```python
from build123d import *

# Parameters (mm, degrees)
SKETCH_1_W             = 25
SKETCH_1_H             = 12
EXTRUDE_1_DEPTH        = 3
SKETCH_2_W             = 8
SKETCH_2_H             = 12
EXTRUDE_2_DEPTH        = 3
FILLET_1_R             = 3
FILLET_2_R             = 1.5
SKETCH_3_R             = 1.6
CUT_EXTRUDE_1_DEPTH    = 3
FILLET_1_OF_MIRROR_1_R = 3
FILLET_2_OF_MIRROR_1_R = 1.5
SKETCH_4_R             = 1.6
CUT_EXTRUDE_2_DEPTH    = 3


with BuildPart() as part:
    # 草图1 → 凸台-拉伸1 (new body)
    with BuildSketch(Plane.XY):
        with Locations((0, -24)):
            Rectangle(SKETCH_1_W, SKETCH_1_H)
    extrude(amount=EXTRUDE_1_DEPTH)

    # 草图2 → 凸台-拉伸2 (add)
    with BuildSketch(Plane.ZY.offset(12.5)):
        with Locations((7, -24)):
            Rectangle(SKETCH_2_W, SKETCH_2_H)
    extrude_2 = extrude(amount=-EXTRUDE_2_DEPTH)

    # 圆角1
    fillet_1_edges = [part.edges().sort_by_distance(p)[0] for p in [
        (-11, -18, 11),
        (-11, -30, 11),
    ]]
    fillet(fillet_1_edges, radius=FILLET_1_R)

    # 圆角2
    fillet_2_edges = [part.edges().sort_by_distance(p)[0] for p in [
        (-9.5, -24, 3),
    ]]
    fillet(fillet_2_edges, radius=FILLET_2_R)

    # 草图3 → 切除-拉伸1 (cut)
    with BuildSketch(Plane.ZY.offset(12.5)):
        with Locations(Location((7, -24, 0), (0, 0, 270))):
            Circle(SKETCH_3_R)
    cut_extrude_1 = extrude(amount=-CUT_EXTRUDE_1_DEPTH, mode=Mode.SUBTRACT)

    # 镜向1: 凸台-拉伸2, 切除-拉伸1 across plane
    add(extrude_2.mirror(Plane(origin=(0, 0, 0), x_dir=(0, 0, 1), z_dir=(1, 0, 0))))
    add(cut_extrude_1.mirror(Plane(origin=(0, 0, 0), x_dir=(0, 0, 1), z_dir=(1, 0, 0))), mode=Mode.SUBTRACT)

    # 圆角1 of 镜向1
    fillet_1_of_mirror_1_edges = [part.edges().sort_by_distance(p)[0] for p in [
        (11, -18, 11),
        (11, -30, 11),
    ]]
    fillet(fillet_1_of_mirror_1_edges, radius=FILLET_1_OF_MIRROR_1_R)

    # 圆角2 of 镜向1
    fillet_2_of_mirror_1_edges = [part.edges().sort_by_distance(p)[0] for p in [
        (9.5, -24, 3),
    ]]
    fillet(fillet_2_of_mirror_1_edges, radius=FILLET_2_OF_MIRROR_1_R)

    # 草图4 → 切除-拉伸2 (cut)
    with BuildSketch(Plane.XY.offset(3)):
        with Locations((5, -24)):
            Circle(SKETCH_4_R)
        with Locations((-5, -24)):
            Circle(SKETCH_4_R)
    extrude(amount=-CUT_EXTRUDE_2_DEPTH, mode=Mode.SUBTRACT)


solid = part.part
```
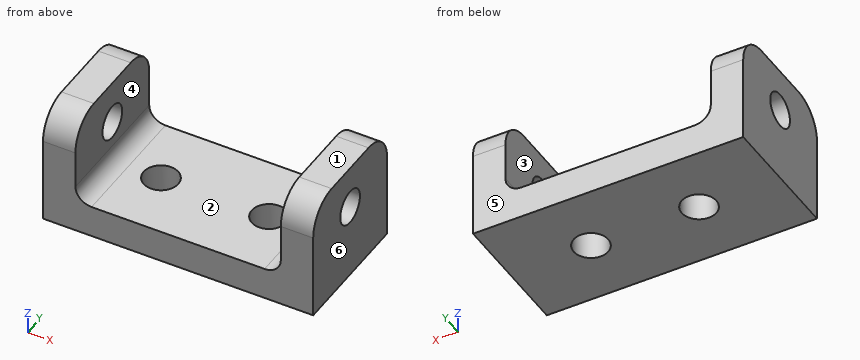
The listing builds one solid part. Answer for the finished solid, in the listing's coordinates (mm). Face numbers are marked on the shaded views. A direction names the side the tool comes from. Give positions to 0.01 mm unless a question says otherwise; leave off trailing zeros. Write each loop counter-clockwise with the first axis right and the second up, starting at its lowest first coordinate (ties: lowest second). Pieces come first, ordered by that corner, then holes. Notation, with made-up numbers: (39, 0) -> (51, 0) arc R15 ccw to (51, 12) -> close; hole circle Ø6 at (53.25, -37). An arc over 180 degrees is marked (long way). Write item = value, one per line. Start each with the question number.
1) Straight lines are drawn through the part: line 1 along Y through (x, z) = (-5, 0.6); line 2 along X through (y, z) = (-24.5, 9); line 3 along Z through (x, y) = (11.25, -24). For each, find the intervals that lie inside material, in ascending order.
2) Determine the mould class of the marked faces 3, 4, 5 and 6 for opening direction X: +X half, -X half, draft (parallel to the pull), parting line (faces both ways), or undercut.
3) Which of the six approach directions +Z, -Z, +X, -X, +Y, -Y give full straight-line access (tool end or side, diameter ignored) to the marked faces 1 and 2?
4) The part is cut by section B-B, the plane x = -5. Determine the outline of the cut face in (y, z), and give its area (3 significant figures).
5) The part is cut by section D-D, the plane x = -1.25. Determine the outline of the cut face in (y, z).
6) Each of these flat-tipped pins is pushed along its axis until it touches: pin 1 (1.9 mm diameter, centred on y = -24, z = 7, fed in from +X); pin 2 (1.5 mm diameter, centred on x = -0.5, y = -27, fed in from +Z). Where does it stop, or does it pass through?
7) The part is cut by section A-A, the plane z = 7. Determine the outline of the cut face in (x, y), and give its area (3 significant figures).
8) The part is cut by section C-C, the plane y = -26.75. Determine the outline of the cut face in (x, z), and give its area (3 significant figures).
Solutions:
q1.line_1 = -30 to -25.6, -22.4 to -18
q1.line_2 = -12.5 to -9.5, 9.5 to 12.5
q1.line_3 = 0 to 5.4, 8.6 to 11
q2.face_3 = undercut
q2.face_4 = undercut
q2.face_5 = draft
q2.face_6 = +X half
q3.face_1 = +Z, +X, -X, +Y, -Y
q3.face_2 = +Z, +Y, -Y
q4.outline = (-30, 0) -> (-25.6, 0) -> (-25.6, 3) -> (-30, 3) -> close; (-22.4, 0) -> (-18, 0) -> (-18, 3) -> (-22.4, 3) -> close
q4.area = 26.4 mm²
q5.outline = (-30, 0) -> (-18, 0) -> (-18, 3) -> (-30, 3) -> close
q6.pin_1 = through
q6.pin_2 = 3
q7.outline = (-12.5, -30) -> (-9.5, -30) -> (-9.5, -25.6) -> (-12.5, -25.6) -> close; (-12.5, -22.4) -> (-9.5, -22.4) -> (-9.5, -18) -> (-12.5, -18) -> close; (9.5, -30) -> (12.5, -30) -> (12.5, -25.6) -> (9.5, -25.6) -> close; (9.5, -22.4) -> (12.5, -22.4) -> (12.5, -18) -> (9.5, -18) -> close
q7.area = 52.8 mm²
q8.outline = (-12.5, 0) -> (12.5, 0) -> (12.5, 11) -> (9.5, 11) -> (9.5, 4.5) arc R1.5 cw to (8, 3) -> (-8, 3) arc R1.5 cw to (-9.5, 4.5) -> (-9.5, 11) -> (-12.5, 11) -> close
q8.area = 124 mm²
